Design review of the part built by this model. Coordinates are the model's own, in mm. Give positions to 0.01 mm unless a question says otherwise; leave off trailing zeros. Write each loop counter-clockwise with the first axis right and the second up, starting at its lowest first coordinate (ties: lowest second). Pieces come first, ordered by that corner, then holes. Notation, with made-up numbers: (27.25, 2) - (75.25, 2) arc R22 cw to (75.25, 32) - close; hole circle Ø8 at (-16.5, 64.25). An arc over 180 degrees is marked (long way). Use a Markdown table: item, result. Add a question column.
Autodesk Inventor part; units mm, degrees
ref_plane "YZ Plane" through (0, 0, 0) normal (1, 0, 0) x (0, 1, 0)
ref_plane "XZ Plane" through (0, 0, 0) normal (0, 1, 0) x (-1, 0, 0)
ref_plane "XY Plane" through (0, 0, 0) normal (0, 0, 1) x (1, 0, 0)
sketch "Sketch3" plane through (0, 0, 0) normal (0, 0, 1) x (1, 0, 0)
  line L0 (0, 0) -> (260, 0)
  line L1 (260, 0) -> (260, 30)
  line L2 (260, 30) -> (-45.1628, 58.3872)
  line L3 (45, 50) -> (45, 0)
  dimension "d11" = 260
  dimension "d12" = 30
  dimension "d13" = 45
  dimension "d14" = 50
extrude "Plate1" add sketch "Sketch3" along normal mid plane 10
fillet "Corner Round1" radius 6 1 edges at (260, 30, 0)
equation "\"d15\" = Thickness"
equation "\"BendReliefDepth\" = 0.5 * Thickness"
properties part number "PRS 940-23 charging hatch reinf 500mm" material "Steel"
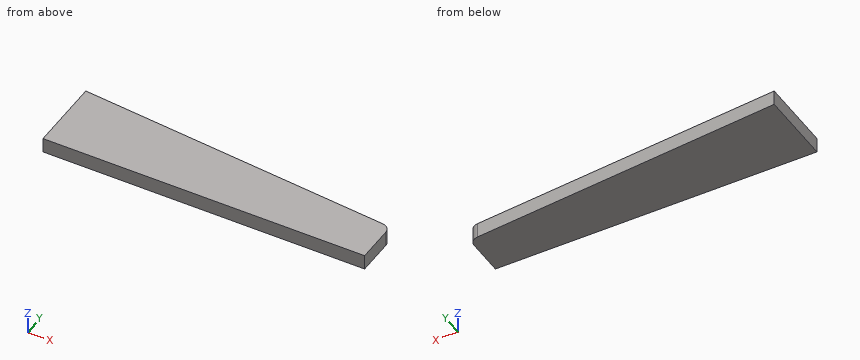
(1) For line 1 along Y through (x, z) = (185.5, 4); line 2 along Y through (x, z) = (129, 2.5); line 3 along X through (y, z) = (28, 0.5), list the stretches that pass through material, from the lowest coordinate up.
(2) Add section B-B (x = 61.5). State the section outline as (y, z) points, and give its area (3 significant figures).
(3) Insertion check: pin 1 (5 mm diameter, centred on x = 230.5, y = 37.5, fed in from +Z). The pin has a flat end and moves straight along its axis. Give the tip position at first contact, or say it passes through.
(4) Add section C-C (y = 34). State the section outline as (x, z) points.
(5) Add section A-A (z = -0.5). State the section outline as (x, y) points.
Answers follow:
| question | item | result |
|---|---|---|
| 1 | line 1 | 0 to 36.93 |
| 1 | line 2 | 0 to 42.19 |
| 1 | line 3 | 45 to 258.9 |
| 2 | outline | (0, -5) - (48.47, -5) - (48.47, 5) - (0, 5) - close |
| 2 | area | 485 mm^2 |
| 3 | pin 1 | through |
| 4 | outline | (45, -5) - (217, -5) - (217, 5) - (45, 5) - close |
| 5 | outline | (45, 0) - (260, 0) - (260, 24.53) arc R6 ccw to (254.56, 30.51) - (45, 50) - close |
